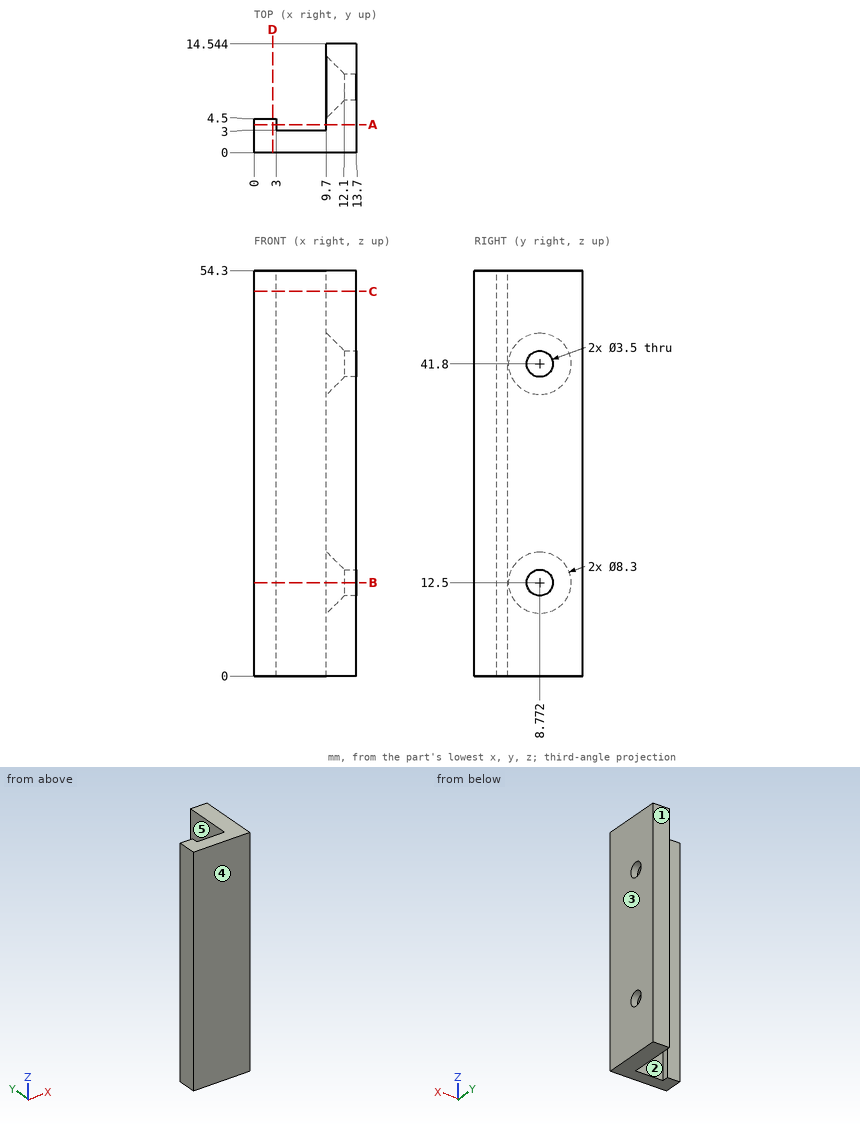
Design review of the part shown in the three views and the two pictorial views. Dimensions are in mm from the part's minimum x, y and z. A direction names the side the tool comes from. Coordinates: 2 decimals unless noted, no trailing zeros. Write each loop counter-clockwise with the first axis right and the second up, starting at its lowest first coordinate (ties: lowest second). Pieces come first, ordered by that corner, then holes. Notation, with made-up numbers: (62, -27) -> (98, -27) arc R22 cw to (98, -3) -> close; hole circle Ø7 at (-12, 29.5). An arc over 180 degrees is marked (long way). Answer in a Markdown table with one row per item.
1. We need section A-A, the plane y = 3.75. State the section outline as (x, z) points, and give its area (3 significant figures).
Answers below:
| item | result |
|---|---|
| outline | (0, 0) -> (3, 0) -> (3, 54.3) -> (0, 54.3) -> close; (9.7, 0) -> (13.7, 0) -> (13.7, 54.3) -> (9.7, 54.3) -> close |
| area | 380 mm^2 |
2. Clearance check with flat-ended pins moving along their axes: pin 1 Ø3 at (y, z) = (8.772, 12.5) entering from -X; pin 2 Ø4 at (y, z) = (8.772, 41.8) entering from -X; pin 3 Ø3.5 at (x, z) = (1, 33) entering from +Y; pin 4 Ø3 at (y, z) = (8.5, 30) entering from -X. State where each tip first meets the part, or that it passes through.
Answers below:
| item | result |
|---|---|
| pin 1 | passes through |
| pin 2 | stops at x = 11.85 |
| pin 3 | stops at y = 4.5 |
| pin 4 | stops at x = 9.7 |
3. We need section D-D, the plane x = 2.5. State the section outline as (y, z) points, and give its area (3 significant figures).
Answers below:
| item | result |
|---|---|
| outline | (0, 0) -> (4.5, 0) -> (4.5, 54.3) -> (0, 54.3) -> close |
| area | 244 mm^2 |
4. Draft analysis for pull direction X (two halves, no side actions). For the marked faces 1, 2 and 3, state which applies: +X half, -X half, draft (parallel to the pull), parting line (faces both ways), or undercut.
Answers below:
| item | result |
|---|---|
| face 1 | draft |
| face 2 | undercut |
| face 3 | +X half |
5. For the marked faces 4 and 5, list the 3-axis set-ups (+Z, -Z, +X, -X, +Y, -Y) from which the entire face can be reached by the end or side of a thin tool; tool diameter is ignored.
Answers below:
| item | result |
|---|---|
| face 4 | +Z, -Z, +X, -X, -Y |
| face 5 | +Z, -Z, +Y |
6. We need section B-B, the plane z = 12.5. State the section outline as (x, y) points, and give its area (3 significant figures).
Answers below:
| item | result |
|---|---|
| outline | (0, 0) -> (13.7, 0) -> (13.7, 7.02) -> (12.1, 7.02) -> (9.7, 4.62) -> (9.7, 3) -> (3, 3) -> (3, 4.5) -> (0, 4.5) -> close; (9.7, 12.92) -> (12.1, 10.52) -> (13.7, 10.52) -> (13.7, 14.54) -> (9.7, 14.54) -> close |
| area | 72.0 mm^2 |
7. We need section C-C, the plane z = 51.5. State the section outline as (x, y) points, and give its area (3 significant figures).
Answers below:
| item | result |
|---|---|
| outline | (0, 0) -> (13.7, 0) -> (13.7, 14.54) -> (9.7, 14.54) -> (9.7, 3) -> (3, 3) -> (3, 4.5) -> (0, 4.5) -> close |
| area | 91.8 mm^2 |
8. Wall thickness on probe 1 along Y at (x, z) = (12.8, 41.8); probe 2 along X at (y, z) = (3.25, 44.5); probe 3 along Y at (x, z) = (8.25, 37): over which ranges is each line inside the solid? List them lowest first. Write a range as [from, to].
Answers below:
| item | result |
|---|---|
| probe 1 | y = [0, 7.02], [10.52, 14.54] |
| probe 2 | x = [0, 3], [9.7, 13.7] |
| probe 3 | y = [0, 3] |
